The model under review builds one solid part; all positions refer to its coordinate system, in mm. Coordinates: 2 decimals unless noted, no trailing zeros. Write each loop counter-clockwise with the first axis right and the second up, starting at its lowest first coordinate (ties: lowest second). Pieces come first, ordered by that corner, then holes.
1) For line 1 (Y direction, x = 83.5, z = 5.2), list the stretches that pass through material, from the lowest coordinate up.
2) Add section A-A, the plane x = 108.5. State the section outline as (y, z) points, then the cut area to 3 significant figures.
3) For P1, Ø3, axis at x = 95, z = 5, coming from the -Y side; P2, Ø1.8, axis at y = 2, z = 3, coming from the +X side; P3, Ø3, axis at y = 3, z = 2, coming from the -X side, all flat-tipped, find the tip position at first contact; note any pin that passes through.
Autodesk Inventor part; units mm, degrees
ref_plane "YZ Plane" through (0, 0, 0) normal (1, 0, 0) x (0, 1, 0)
ref_plane "XZ Plane" through (0, 0, 0) normal (0, 1, 0) x (-1, 0, 0)
ref_plane "XY Plane" through (0, 0, 0) normal (0, 0, 1) x (1, 0, 0)
sketch "Sketch1" plane through (0, 0, 0) normal (0, 0, 1) x (1, 0, 0)
  line L0 (0, 6) -> (120, 6)
  line L1 (120, 6) -> (120, 0)
  line L2 (120, 0) -> (0, 0)
  line L3 (0, 0) -> (0, 6)
  line L4 (3, 6) -> (3, 0)
  line L5 (9, 6) -> (9, 0)
  line L6 (9, 6) -> (9, 0)
  line L7 (15, 6) -> (15, 0)
  line L8 (15, 6) -> (15, 0)
  line L9 (21, 6) -> (21, 0)
  line L10 (21, 6) -> (21, 0)
  line L11 (27, 6) -> (27, 0)
  line L12 (27, 6) -> (27, 0)
  line L13 (33, 6) -> (33, 0)
  line L14 (33, 6) -> (33, 0)
  line L15 (39, 6) -> (39, 0)
  line L16 (39, 6) -> (39, 0)
  line L17 (45, 6) -> (45, 0)
  line L18 (45, 6) -> (45, 0)
  line L19 (51, 6) -> (51, 0)
  line L20 (51, 6) -> (51, 0)
  line L21 (57, 6) -> (57, 0)
  line L22 (57, 6) -> (57, 0)
  line L23 (63, 6) -> (63, 0)
  line L24 (63, 6) -> (63, 0)
  line L25 (69, 6) -> (69, 0)
  line L26 (69, 6) -> (69, 0)
  line L27 (75, 6) -> (75, 0)
  line L28 (75, 6) -> (75, 0)
  line L29 (81, 6) -> (81, 0)
  line L30 (81, 6) -> (81, 0)
  line L31 (87, 6) -> (87, 0)
  line L32 (87, 6) -> (87, 0)
  line L33 (93, 6) -> (93, 0)
  line L34 (93, 6) -> (93, 0)
  line L35 (99, 6) -> (99, 0)
  line L36 (99, 6) -> (99, 0)
  line L37 (105, 6) -> (105, 0)
  line L38 (105, 6) -> (105, 0)
  line L39 (111, 6) -> (111, 0)
  line L40 (111, 6) -> (111, 0)
  line L41 (117, 6) -> (117, 0)
  line L42 (0, 6) -> (0, 126)
  line L43 (120, 6) -> (120, 126)
  line L44 (120, 126) -> (0, 126)
  point P0 (0, 3)
  point P1 (3, 3)
  point P2 (9, 3)
  point P3 (15, 3)
  point P4 (21, 3)
  point P5 (27, 3)
  point P6 (33, 3)
  point P7 (39, 3)
  point P8 (45, 3)
  point P9 (51, 3)
  point P10 (57, 3)
  point P11 (63, 3)
  point P12 (69, 3)
  point P13 (75, 3)
  point P14 (81, 3)
  point P15 (87, 3)
  point P16 (93, 3)
  point P17 (99, 3)
  point P18 (105, 3)
  point P19 (111, 3)
  dimension "d4" = 120
  dimension "d5" = 6
  dimension "d6" = 3
  dimension "d7" = 6
  dimension "d8" = 6
  dimension "d10" = 120
  dimension "d11" = 120
extrude "Extrusion1" add sketch "Sketch1" along normal blind 6 contours L42 L44 L43 L0 | L0 L5 L2 L4 | L0 L9 L2 L7 | L41 L2 L39 L0 | L0 L13 L2 L11 | L37 L2 L35 L0 | L0 L17 L2 L15 | L33 L2 L31 L0 | L0 L21 L2 L19 | L29 L2 L27 L0 | L0 L25 L2 L23
properties part number "wall inteface V1"
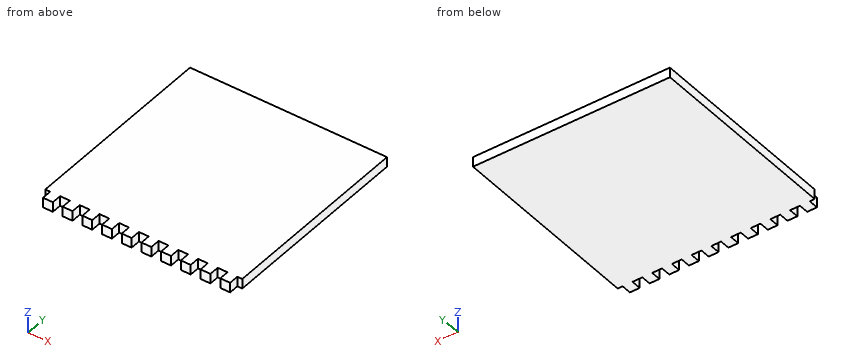
Geometry results:
1. line 1: y = 6 to 126
2. outline: (6, 0) - (126, 0) - (126, 6) - (6, 6) - close
2. area: 720 mm2
3. P1: stops at y = 6
3. P2: stops at x = 117
3. P3: stops at x = 3
